from build123d import *

# Parameters (mm, degrees)
EXTRUDE_1_DEPTH     = 10
SKETCH_2_R          = 8
EXTRUDE_2_DEPTH     = 50
SKETCH_3_R          = 4
CUT_EXTRUDE_2_DEPTH = 15


with BuildPart() as part:
    # 草图1 → 凸台-拉伸1 (new body)
    with BuildSketch(Plane.XY):
        Polygon((15, 0), (7.5, 12.990381057), (-7.5, 12.990381057), (-15, 0), (-7.5, -12.990381057), (7.5, -12.990381057), align=None)
    extrude(amount=EXTRUDE_1_DEPTH)

    # 草图2 → 凸台-拉伸2 (add)
    with BuildSketch(Plane.XY):
        Circle(SKETCH_2_R)
    extrude(amount=EXTRUDE_2_DEPTH)

    # 草图3 → 切除-拉伸2 (cut)
    with BuildSketch(Plane.XY):
        Circle(SKETCH_3_R)
    extrude(amount=CUT_EXTRUDE_2_DEPTH, mode=Mode.SUBTRACT)


solid = part.part
Geometry check sheet. Reference: the model listing, model coordinates, mm. A direction names the side the tool comes from. Give positions to 0.01 mm unless a question says otherwise; leave off trailing zeros. Write each loop counter-clockwise with the first axis right and the second up, starting at its lowest first coordinate (ties: lowest second). Pieces come first, ordered by that corner, then holes.
1) Release check for a two-part mould opening along Y. For faces 4 (the face through (0, 0, 15)), 5 (the face through (-11.302, -6.404, 4.93)), 6 (the face through (3, 3, 0)) record: released by +Y, released by -Y, zero draft, split by the parting line, or undercut.
Values follow:
face 4: undercut
face 5: released by -Y
face 6: zero draft
2) Set-up check for faces 1 (the face through (0, 12.99, 5)), 2 (the face through (-0.867, -3.905, 7.395)), 3 (the face through (6, 6, 10)): record each of +Z, -Z, +X, -X, +Y, -Y from which the full face is reachable in a straight line by a thin tool's end or side.
Values follow:
face 1: +Z, -Z, +X, -X, +Y
face 2: -Z
face 3: +Z
3) Cross-section at B-B (x = 0). Record the boundary of the cut face in (y, z), plus the area to 3 significant figures.
Values follow:
outline: (-12.99, 0) - (-4, 0) - (-4, 15) - (4, 15) - (4, 0) - (12.99, 0) - (12.99, 10) - (8, 10) - (8, 50) - (-8, 50) - (-8, 10) - (-12.99, 10) - close
area: 780 mm2
4) Thickness scan on line 1 (Y direction, x = 0, z = 8.5); line 2 (Z direction, x = -12, y = -3.75); line 3 (Y direction, x = 1.5, z = 11). Record the ranges inside material, lowest first.
Values follow:
line 1: y = -12.99 to -4, 4 to 12.99
line 2: z = 0 to 10
line 3: y = -7.86 to -3.71, 3.71 to 7.86
5) Go/stop test with flat-tipped pins: pin 1 Ø2.5 at (x, y) = (0.5, 1) entering from -Z; pin 2 Ø2 at (y, z) = (7, 44.5) entering from -X; pin 3 Ø3 at (x, y) = (-10.5, -4) entering from +Z. Record where each tip stops, or that it passes through.
Values follow:
pin 1: stops at z = 15
pin 2: stops at x = -5.29
pin 3: stops at z = 10
6) Cross-section at A-A (z = 8). Record the boundary of the cut face in (x, y).
Values follow:
outline: (-15, 0) - (-7.5, -12.99) - (7.5, -12.99) - (15, 0) - (7.5, 12.99) - (-7.5, 12.99) - close; hole circle Ø8 at (0, 0)
7) Cross-section at C-C (y = 1.75). Record the boundary of the cut face in (x, z).
Values follow:
outline: (-13.99, 0) - (-3.6, 0) - (-3.6, 15) - (3.6, 15) - (3.6, 0) - (13.99, 0) - (13.99, 10) - (7.81, 10) - (7.81, 50) - (-7.81, 50) - (-7.81, 10) - (-13.99, 10) - close
8) Cross-section at D-D (z = 42.5). Record the boundary of the cut face in (x, y).
Values follow:
outline: circle Ø16 at (0, 0)
